from build123d import *

# Parameters (mm, degrees)
SKETCH1_R           = 10
BOSS_EXTRUDE1_DEPTH = 90


with BuildPart() as part:
    # Sketch1 → Boss-Extrude1 (new body)
    with BuildSketch(Plane.XY):
        with BuildLine():
            Line((60, 40), (90, 40))
            Line((90, 40), (90, -20))
            ThreePointArc((90, -20), (84.142135624, -34.142135624), (70, -40))
            Line((70, -40), (60, -40))
            Line((60, -40), (60, -35))
            ThreePointArc((60, -35), (58.535533906, -31.464466094), (55, -30))
            Line((55, -30), (-55, -30))
            ThreePointArc((-55, -30), (-58.535533906, -31.464466094), (-60, -35))
            Line((-60, -35), (-60, -40))
            Line((-60, -40), (-70, -40))
            ThreePointArc((-70, -40), (-84.142135624, -34.142135624), (-90, -20))
            Line((-90, -20), (-90, 40))
            Line((-90, 40), (-60, 40))
            ThreePointArc((-60, 40), (0, -20), (60, 40))
        make_face()
        with Locations(Location((-70, -20, 0), (0, 0, 180))):
            Circle(SKETCH1_R, mode=Mode.SUBTRACT)
        with Locations(Location((70, -20, 0), (0, 0, 180))):
            Circle(SKETCH1_R, mode=Mode.SUBTRACT)
    extrude(amount=BOSS_EXTRUDE1_DEPTH)


solid = part.part
Could you check a few things on this model? Use its own coordinates, in mm. A direction names the side the tool comes from. Coordinates: 2 decimals unless noted, no trailing zeros. Order: outer loops, then holes, each group sorted by start corner. A loop starts at its lowest first (then second) coordinate and runs counter-clockwise, first axis right, second up.
Q1. Please list where these lines run through material, in increasing order: L1, parallel to Y at x = 70, z = 26; L2, parallel to X at y = -28.5, z = 42.5; L3, parallel to X at y = -31, z = 6.
Q2. Will these pins go through, and if not, where does the flat tip stop? pin 1 (18 mm diameter, centred on x = -70, y = -20, fed in from +Z); pin 2 (4 mm diameter, centred on y = -37, z = 41.5, fed in from +X); pin 3 (3 mm diameter, centred on x = 40.5, z = 50, fed in from +Y); pin 4 (12 mm diameter, centred on x = -17.5, z = 19.5, fed in from -Y).
Q3. Suppose I cut it at D-D on x = -46. Please give me the cut outline in (y, z).
Q4. Suppose I cut it at C-C on x = 0. Please give me the cut outline in (y, z), and give its area (3 significant figures).
Q5. Thinking about a two-plate mould opening in X: for faces 1 (the flat face through (65, -40, 44)), 2 (the flat face through (-90, 10, 44)), 3 (the cylindrical face through (-60, -20, 44)), which applies, released by +X, released by -X, zero draft, split by the parting line, or undercut?
Q6. Which directions (+Z, -Z, +X, -X, +Y, -Y) give clear straight access to the entire face, cutting with the end or side of a thin tool? Please do faces 4 (the cylindrical face through (80, -20, 44)), 5 (the flat face through (1, -30, 44)).
Q7. Suppose I cut it at A-A on z = 50. Please give me the cut outline in (x, y), and give its area (3 significant figures).
Q8. Suppose I cut it at B-B on y = 7.5. Please give me the cut outline in (x, z).
Answer:
1. L1: y = -40 to -30, -10 to 40
1. L2: x = -88.1 to -75.27, -64.73 to 64.73, 75.27 to 88.1
1. L3: x = -86.7 to -58, 58 to 86.7
2. pin 1: passes through
2. pin 2: stops at x = 83.23
2. pin 3: stops at y = -2.85
2. pin 4: stops at y = -30
3. outline: (-30, 0) - (1.48, 0) - (1.48, 90) - (-30, 90) - close
4. outline: (-30, 0) - (-20, 0) - (-20, 90) - (-30, 90) - close
4. area: 900 mm2
5. face 1: zero draft
5. face 2: released by -X
5. face 3: undercut
6. face 4: +Z, -Z
6. face 5: +Z, -Z, -Y
7. outline: (-90, -20) arc R20 ccw to (-70, -40) - (-60, -40) - (-60, -35) arc R5 cw to (-55, -30) - (55, -30) arc R5 cw to (60, -35) - (60, -40) - (70, -40) arc R20 ccw to (90, -20) - (90, 40) - (60, 40) arc R60 cw to (-60, 40) - (-90, 40) - close; hole circle Ø20 at (-70, -20); hole circle Ø20 at (70, -20)
7. area: 6,760 mm2
8. outline: (-90, 0) - (-50.44, 0) - (-50.44, 90) - (-90, 90) - close; (50.44, 0) - (90, 0) - (90, 90) - (50.44, 90) - close
